```python
from build123d import *

# Parameters (mm, degrees)
SKETCH1_R  = 3
HEAD_DEPTH = 9
SKETCH2_R  = 0.5
PINS_DEPTH = 18


with BuildPart() as part:
    # Sketch1 → Head (new body)
    with BuildSketch(Plane(origin=(0, 0, 0), x_dir=(1, 0, 0), z_dir=(0, 1, 0))):
        with Locations(Location((0, 0, 0), (0, 0, 270))):
            Circle(SKETCH1_R)
    extrude(amount=-HEAD_DEPTH)

    # Sketch2 → Pins (add)
    with BuildSketch(Plane(origin=(0, 0, 0), x_dir=(1, 0, 0), z_dir=(0, 1, 0))):
        with Locations(Location((-1, 0, 0), (0, 0, 270))):
            Circle(SKETCH2_R)
        with Locations(Location((1, 0, 0), (0, 0, 270))):
            Circle(SKETCH2_R)
    extrude(amount=PINS_DEPTH)


solid = part.part
```
Verification items for the finished model (mm, model axes). A direction names the side the tool comes from. Coordinates: 2 decimals unless noted, no trailing zeros. Write each loop counter-clockwise with the first axis right and the second up, starting at its lowest first coordinate (ties: lowest second). Pieces come first, ordered by that corner, then holes. Notation, with made-up numbers: M -10.5,89 L 37.5,89 A27 cw 37.5,118 Z; hole C 89,-36.75 d6. An arc over 180 degrees is marked long. Answer as a JSON object with one key per item and string values. Group by question number.
(1) Release check for a two-part mould opening along X. For faces 3 (the face through (0.9, -4.44, 2.86)), 4 (the face through (0.512, 8.874, -0.108)), 5 (the face through (-1, 18, 0)) record: +X half, -X half, draft (parallel to the pull), parting line (faces both ways), or undercut.
(2) Cross-section at D-D, the plane x = 2.4. Record the cut outline in (y, z).
(3) Cross-section at C-C, the plane z = 0. Record the cut outline in (x, y), and give its area (3 significant figures).
(4) Cross-section at A-A, the plane y = 14.25. Record the cut outline in (x, z).
(5) Material ranges on line 1 (Y direction, x = -0.1, z = 2.6); line 2 (X direction, y = 0.75, z = 0.2); line 3 (Z direction, x = -1.75, y = -0.5), recorded low to high.
(6) Cross-section at B-B, the plane x = -1. Record the cut outline in (y, z), and give its area (3 significant figures).
(7) Tool access check on faces 1 (the face through (1, 18, 0)), 2 (the face through (-1.3, 8.9, -0.4)). Record the directions out of +Z, -Z, +X, -X, +Y, -Y that give a thin tool (end or side, any length) a straight path to the whole face; none if there is none.
Reply:
{
 "1": {"face 3": "parting line", "face 4": "undercut", "face 5": "draft"},
 "2": {"outline": "M -9,-1.8 L 0,-1.8 L 0,1.8 L -9,1.8 Z"},
 "3": {"outline": "M -3,-9 L 3,-9 L 3,0 L 1.5,0 L 1.5,18 L 0.5,18 L 0.5,0 L -0.5,0 L -0.5,18 L -1.5,18 L -1.5,0 L -3,0 Z", "area": "90.0 mm²"},
 "4": {"outline": "C -1,0 d1; C 1,0 d1"},
 "5": {"line 1": "-9 to 0", "line 2": "-1.46 to -0.54, 0.54 to 1.46", "line 3": "-2.44 to 2.44"},
 "6": {"outline": "M -9,-2.83 L 0,-2.83 L 0,-0.5 L 18,-0.5 L 18,0.5 L 0,0.5 L 0,2.83 L -9,2.83 Z", "area": "68.9 mm²"},
 "7": {"face 1": "+Z, -Z, +X, -X, +Y", "face 2": "+Y"}
}
